Verification items for this drawing (mm, ordinates from the low corner). Give positions to 0.01 mm unless a question says otherwise; leave off trailing zeros. Order: outer loops, then holes, each group sorted by start corner. A loop starts at its lowest first (then second) coordinate and runs counter-clockwise, first axis right, second up. Notation, with made-up numbers: M 65,57.5 L 116,57.5 A12 cw 116,70.5 Z; hole C 71,-38.75 d5. An arc over 180 degrees is marked long. Answer as a JSON object with one key per item and string values.
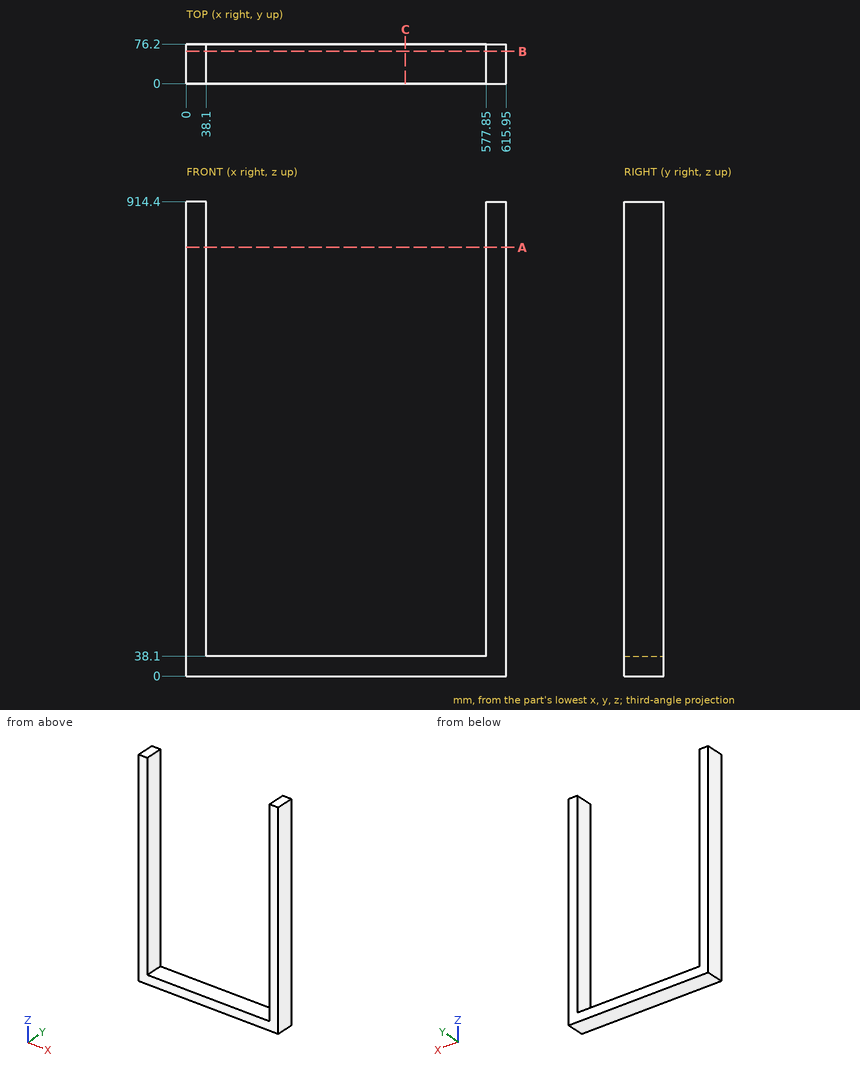
Q1. Material ranges on L1, parallel to X at y = 15, z = 283.5; L2, parallel to Z at x = 485, y = 33, recorded low to high.
Resolved:
{"L1": "x = 0 to 38.1, 577.85 to 615.95", "L2": "z = 0 to 38.1"}
Q2. Section check B-B on y = 62. Record the cut outline in (x, z), then the cut area to 3 significant figures.
Resolved:
{"outline": "M 0,0 L 615.95,0 L 615.95,914.4 L 577.85,914.4 L 577.85,38.1 L 38.1,38.1 L 38.1,914.4 L 0,914.4 Z", "area": "90,200 mm²"}
Q3. Section check A-A on z = 826. Record the cut outline in (x, y), then the cut area to 3 significant figures.
Resolved:
{"outline": "M 0,0 L 38.1,0 L 38.1,76.2 L 0,76.2 Z; M 577.85,0 L 615.95,0 L 615.95,76.2 L 577.85,76.2 Z", "area": "5,810 mm²"}
Q4. Gauge pin test, flat ends, axial feed: pin 1 Ø6 at (x, y) = (114.5, 67) entering from -Z; pin 2 Ø1 at (x, y) = (318, 49.5) entering from +Z. Record the tip position at first contact, or that the pin passes through.
Resolved:
{"pin 1": "stops at z = 0", "pin 2": "stops at z = 38.1"}
Q5. Section check C-C on x = 422. Record the cut outline in (y, z), then the cut area to 3 significant figures.
Resolved:
{"outline": "M 0,0 L 76.2,0 L 76.2,38.1 L 0,38.1 Z", "area": "2,900 mm²"}
